from build123d import *

# Parameters (mm, degrees)
F1_R     = 3
F2_DEPTH = 40
F3_T     = -3
F4_R     = 3


with BuildPart() as f2:
    # F1 (on Front) → F2 (new body)
    with BuildSketch(Plane.XZ):
        Polygon((42.5, 37.0096189432), (20, 50), (20, 110), (-20, 110), (-20, 50), (-42.5, 37.0096189432), (-42.5, -50), (42.5, -50), align=None)
        Circle(F1_R, mode=Mode.SUBTRACT)
    extrude(amount=F2_DEPTH)

    # F3
    f3_openings = [f2.faces().sort_by_distance(p)[0] for p in [
        (0, -40, 16.88666),
    ]]
    offset(amount=F3_T, openings=f3_openings, kind=Kind.INTERSECTION)

    # F4
    f4_edges = [f2.edges().sort_by_distance(p)[0] for p in [
        (39.5, -3, -5.861216),
        (0, -3, -47),
        (-39.5, -3, -5.861216),
        (17, -3, 77.633975),
        (0, -3, 107),
        (-17, -3, 77.633975),
        (-20, -20, 110),
        (20, -20, 110),
        (42.5, -20, -50),
        (-42.5, -20, -50),
        (0, 0, 110),
        (20, 0, 80),
        (-42.5, 0, -6.495191),
        (-20, 0, 80),
        (0, 0, -50),
        (42.5, 0, -6.495191),
        (-6, -3, 0),
        (42.5, -20, 37.009619),
        (20, -20, 50),
        (31.25, 0, 43.504809),
        (-20, -20, 50),
        (-42.5, -20, 37.009619),
        (-31.25, 0, 43.504809),
    ]]
    fillet(f4_edges, radius=F4_R)


solid = f2.part
Verification items for the finished model (mm, model axes). A direction names the side the tool comes from. Coordinates: 2 decimals unless noted, no trailing zeros. Order: outer loops, then holes, each group sorted by start corner. A loop starts at its lowest first (then second) coordinate and runs counter-clockwise, first axis right, second up.
1. Sectioned sample at C-C, the plane z = 0. Record the cut outline in (x, y), and give its area (3 significant figures).
Results found:
outline: (-42.5, -40) - (-39.5, -40) - (-39.5, -6) arc R3 cw to (-36.5, -3) - (-9, -3) arc R3 cw to (-6, -6) - (-6, -40) - (-3, -40) - (-3, 0) - (-39.5, 0) arc R3 ccw to (-42.5, -3) - close; (3, -40) - (6, -40) - (6, -6) arc R3 cw to (9, -3) - (36.5, -3) arc R3 cw to (39.5, -6) - (39.5, -40) - (42.5, -40) - (42.5, -3) arc R3 ccw to (39.5, 0) - (3, 0) - close
area: 685 mm2
2. Sectioned sample at A-A, the plane y = -33. Record the cut outline in (x, z).
Results found:
outline: (-42.5, -47) arc R3 ccw to (-39.5, -50) - (39.5, -50) arc R3 ccw to (42.5, -47) - (42.5, 35.28) arc R3 ccw to (41, 37.88) - (21.5, 49.13) arc R3 cw to (20, 51.73) - (20, 107) arc R3 ccw to (17, 110) - (-17, 110) arc R3 ccw to (-20, 107) - (-20, 51.73) arc R3 cw to (-21.5, 49.13) - (-41, 37.88) arc R3 ccw to (-42.5, 35.28) - close; circle Ø12 at (0, 0); hole (-39.5, -47) - (39.5, -47) - (39.5, 35.28) - (17, 48.27) - (17, 107) - (-17, 107) - (-17, 48.27) - (-39.5, 35.28) - close; hole circle Ø6 at (0, 0)
3. Sectioned sample at B-B, the plane x = 0. Record the cut outline in (y, z), and give its area (3 significant figures).
Results found:
outline: (-40, -50) - (-3, -50) arc R3 ccw to (0, -47) - (0, -3) - (-40, -3) - (-40, -6) - (-6, -6) arc R3 cw to (-3, -9) - (-3, -44) arc R3 cw to (-6, -47) - (-40, -47) - close; (-40, 3) - (0, 3) - (0, 107) arc R3 ccw to (-3, 110) - (-40, 110) - (-40, 107) - (-6, 107) arc R3 cw to (-3, 104) - (-3, 9) arc R3 cw to (-6, 6) - (-40, 6) - close
area: 910 mm2
4. Go/stop test with flat-tipped pins: pin 1 Ø17 at (y, z) = (-14.5, 76.5) entering from +X; pin 2 Ø2 at (x, z) = (-12, -33.5) entering from -Y; pin 3 Ø12 at (y, z) = (-29.5, 52.5) entering from +X; pin 4 Ø5 at (x, z) = (0, 0) entering from -Y. Record where each tip stops, or that it passes through.
Results found:
pin 1: stops at x = 20
pin 2: stops at y = -3
pin 3: stops at x = 26.06
pin 4: passes through
5. Set-up check for faces 4 (the face through (-1, -3, 15)), 5 (the face through (-3, -20, 0)), 6 (the face through (19.14, -0.9, 79.75)), 7 (the face through (20, -21, 79)): record each of +Z, -Z, +X, -X, +Y, -Y from which the full face is reachable in a straight line by a thin tool's end or side.
Results found:
face 4: -Y
face 5: +Y, -Y
face 6: +Z, +X, +Y
face 7: +Z, +X, +Y, -Y
6. Release check for a two-part mould opening along Z. For faces 1 (the face through (-19.1, -21.76, 109.14)), 2 (the face through (-16.14, -3.9, 77.22)), 3 (the face through (42.5, -21, -6)) record: +Z half, -Z half, draft (parallel to the pull), parting line (faces both ways), or undercut.
Results found:
face 1: +Z half
face 2: undercut
face 3: draft
7. Scan lines: line 1 (Z direction, x = 0, y = -26.5); line 2 (X direction, y = -20, z = 98); line 3 (X direction, y = -9, z = 10). Record each from-to range of solid material in increasing order.
Results found:
line 1: z = -50 to -47, -6 to -3, 3 to 6, 107 to 110
line 2: x = -20 to -17, 17 to 20
line 3: x = -42.5 to -39.5, 39.5 to 42.5
8. Sectioned sample at D-D, the plane z = 57. Record the cut outline in (x, y).
Results found:
outline: (-20, -40) - (-17, -40) - (-17, -6) arc R3 cw to (-14, -3) - (14, -3) arc R3 cw to (17, -6) - (17, -40) - (20, -40) - (20, -3) arc R3 ccw to (17, 0) - (-17, 0) arc R3 ccw to (-20, -3) - close
